from build123d import *

# Parameters (mm, degrees)
F0_W     = 10
F0_H     = 138
F0_W_2   = 4.659399
F0_H_2   = 28.3
F0_W_3   = 4.6
F1_DEPTH = 11.95
F2_DEPTH = 9


with BuildPart() as f1:
    # F0 (on Front) → F1 (new body)
    with BuildSketch(Plane.XZ):
        with Locations((-25.254509, -12.323071)):
            Rectangle(F0_W, F0_H)
        with Locations((-25.291808, -60.673071)):
            Rectangle(F0_W_2, F0_H_2, mode=Mode.SUBTRACT)
        Polygon((-27.562109, -41.183438), (-27.562109, -14.323071), (-22.962109, -14.323071), (-22.962109, -42.623071), (-27.562109, -42.623071), align=None, mode=Mode.SUBTRACT)
        with Locations((-25.262109, 3.726929)):
            Rectangle(F0_W_3, F0_H_2, mode=Mode.SUBTRACT)
        with Locations((-25.262109, 35.926929)):
            Rectangle(F0_W_3, F0_H_2, mode=Mode.SUBTRACT)
        with Locations((-25.262109, 35.926929)):
            Rectangle(F0_W_3, F0_H_2)
        with Locations((-25.262109, 3.726929)):
            Rectangle(F0_W_3, F0_H_2)
        Polygon((-22.962109, -14.323071), (-27.562109, -14.323071), (-27.562109, -41.183438), (-27.562109, -42.623071), (-22.962109, -42.623071), align=None)
        with Locations((-25.291808, -60.673071)):
            Rectangle(F0_W_2, F0_H_2)
    extrude(amount=F1_DEPTH)

    # F0 (on Front) → F2 (cut)
    with BuildSketch(Plane.XZ):
        with Locations((-25.262109, 35.926929)):
            Rectangle(F0_W_3, F0_H_2)
        with Locations((-25.262109, 3.726929)):
            Rectangle(F0_W_3, F0_H_2)
        Polygon((-22.962109, -14.323071), (-27.562109, -14.323071), (-27.562109, -41.183438), (-27.562109, -42.623071), (-22.962109, -42.623071), align=None)
        with Locations((-25.291808, -60.673071)):
            Rectangle(F0_W_2, F0_H_2)
    extrude(amount=F2_DEPTH, mode=Mode.SUBTRACT)

    # F3: F1 across face


with BuildPart() as f1_1:
    add(f1.part)
    add(f1.part.mirror(Plane(origin=(-25.254509, -11.95, -12.323071), x_dir=(1, 0, 0), z_dir=(0, -1, 0))))


solid = f1_1.part
Read the model definition and answer for the solid it produces. Units are mm, in the model's axes. A direction names the side the tool comes from. Give positions to 0.01 mm unless a question says otherwise; leave off trailing zeros. Write each loop counter-clockwise with the first axis right and the second up, starting at its lowest first coordinate (ties: lowest second). Pieces come first, ordered by that corner, then holes. Notation, with made-up numbers: (-17, 5) -> (2, 5) arc R34 ccw to (2, 35) -> close; hole circle Ø6 at (17.25, -19). An arc over 180 degrees is marked (long way). Answer as a JSON object with one key per item and string values. Group by question number.
1) Find section B-B (z = -41). Write down the section's boundary in (x, y).
2) A tool of negligible diameter and unlimited length cuts with its end or side. For faces 1 (the flat face through (-22.962, -19, 36)), 2 (the flat face through (-25, -12, -81.323)), 3 (the flat face through (-27.562, -4, -28)), from which of +Z, -Z, +X, -X, +Y, -Y can it reach the whole face along a straight path? Write none if from no direction.
3) This flat-tipped pin is pushed along its axis until it touches: P1, Ø3.5, axis at x = -25.5, z = 35.5, coming from the -Y side. Where does it stop, or does it pass through?
4) Consider L1, parallel to Z at x = -24.5, y = -18.5; L2, parallel to X at y = -22.5, z = -5; L3, parallel to Y at x = -25, z = -69. Determine where each line is inside the solid, lowest interval first. Write a range as from..to.
5) Find section A-A (y = -21). Write down the section's boundary in (x, z), and give its area (3 significant figures).
6) The mould has two halves that part along X. Classify faces 4 (the flat face through (-20.255, -12, -13)), 5 (the flat face through (-25, -14.9, 4)), 6 (the flat face through (-25, -23.9, -11)): +X half, -X half, draft (parallel to the pull), parting line (faces both ways), or undercut.
Values follow:
{
 "1": {"outline": "(-30.25, -23.9) -> (-27.56, -23.9) -> (-27.56, -14.9) -> (-22.96, -14.9) -> (-22.96, -23.9) -> (-20.25, -23.9) -> (-20.25, 0) -> (-22.96, 0) -> (-22.96, -9) -> (-27.56, -9) -> (-27.56, 0) -> (-30.25, 0) -> close"},
 "2": {"face 1": "-Y", "face 2": "-Z, +X, -X, +Y, -Y", "face 3": "+Y"},
 "3": {"P1": "stops at y = -14.9"},
 "4": {"L1": "z = -81.32..-74.82, -46.52..-42.62, -14.32..-10.42, 17.88..21.78, 50.08..56.68", "L2": "x = -30.25..-27.56, -22.96..-20.25", "L3": "y = -14.9..-9"},
 "5": {"outline": "(-30.25, -81.32) -> (-20.25, -81.32) -> (-20.25, 56.68) -> (-30.25, 56.68) -> close; hole (-27.62, -74.82) -> (-22.96, -74.82) -> (-22.96, -46.52) -> (-27.62, -46.52) -> close; hole (-27.56, -42.62) -> (-22.96, -42.62) -> (-22.96, -14.32) -> (-27.56, -14.32) -> close; hole (-27.56, -10.42) -> (-22.96, -10.42) -> (-22.96, 17.88) -> (-27.56, 17.88) -> close; hole (-27.56, 21.78) -> (-22.96, 21.78) -> (-22.96, 50.08) -> (-27.56, 50.08) -> close", "area": "858 mm2"},
 "6": {"face 4": "+X half", "face 5": "undercut", "face 6": "draft"}
}
